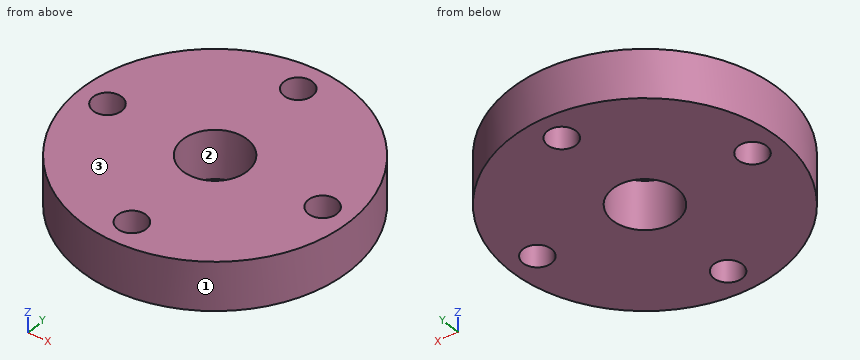
```python
from build123d import *

# Parameters (mm, degrees)
SKETCH1_R           = 16.4
SKETCH1_R_2         = 4
SKETCH1_R_3         = 1.8
BOSS_EXTRUDE1_DEPTH = 6
MOVE_FACE1_BY       = 0.05
MOVE_FACE1_2_BY     = 0.05
MOVE_FACE1_3_BY     = 0.05
MOVE_FACE1_4_BY     = 0.05
MOVE_FACE1_5_BY     = 0.05
MOVE_FACE1_6_BY     = 0.05


with BuildPart() as part:
    # Sketch1 → Boss-Extrude1 (new body)
    with BuildSketch(Plane.XY):
        Circle(SKETCH1_R)
        Circle(SKETCH1_R_2, mode=Mode.SUBTRACT)
        with Locations((0, 13)):
            Circle(SKETCH1_R_3, mode=Mode.SUBTRACT)
        with Locations((13, 0)):
            Circle(SKETCH1_R_3, mode=Mode.SUBTRACT)
        with Locations((0, -13)):
            Circle(SKETCH1_R_3, mode=Mode.SUBTRACT)
        with Locations((-13, 0)):
            Circle(SKETCH1_R_3, mode=Mode.SUBTRACT)
    extrude(amount=BOSS_EXTRUDE1_DEPTH)

    # Move Face1: a curved face moved outward by 0.05
    add(Solid.thicken(part.faces().sort_by_distance((-1.8, 13, 3))[0], MOVE_FACE1_BY))

    # Move Face1 2: a curved face moved outward by 0.05
    add(Solid.thicken(part.faces().sort_by_distance((-16.4, 0, 3))[0], MOVE_FACE1_2_BY))

    # Move Face1 3: a curved face moved outward by 0.05
    add(Solid.thicken(part.faces().sort_by_distance((-4, 0, 3))[0], MOVE_FACE1_3_BY))

    # Move Face1 4: a curved face moved outward by 0.05
    add(Solid.thicken(part.faces().sort_by_distance((11.2, 0, 3))[0], MOVE_FACE1_4_BY))

    # Move Face1 5: a curved face moved outward by 0.05
    add(Solid.thicken(part.faces().sort_by_distance((-1.8, -13, 3))[0], MOVE_FACE1_5_BY))

    # Move Face1 6: a curved face moved outward by 0.05
    add(Solid.thicken(part.faces().sort_by_distance((-14.8, 0, 3))[0], MOVE_FACE1_6_BY))


solid = part.part
```
Design review of the part built by this model. Coordinates are the model's own, in mm. Face numbers are marked on the shaded views. Coordinates: 2 decimals unless noted, no trailing zeros. Order: outer loops, then holes, each group sorted by start corner. A loop starts at its lowest first (then second) coordinate and runs counter-clockwise, first axis right, second up. Notation, with made-up numbers: (-32, 76.5) - (26, 76.5) arc R26 cw to (26, 97.5) - close; hole circle Ø10 at (-29.75, 6.5). An arc over 180 degrees is marked (long way). Answer in a Markdown table with one row per item.
(1) The part is to be moulded in two halves that separate along Y. For the marked faces 1, 2 and 3, say which applies: released by +Y, released by -Y, zero draft, split by the parting line, or undercut.
Checked values:
| item | result |
|---|---|
| face 1 | split by the parting line |
| face 2 | undercut |
| face 3 | zero draft |
(2) Clearance check with flat-ended pins moving along their axes: pin 1 (3 mm diameter, centred on x = 3, y = 3.5, fed in from -Z); pin 2 (1.5 mm diameter, centred on y = -12, z = 4, fed in from -X); pin 3 (3 mm diameter, centred on x = 0, y = 13, fed in from -Z); pin 4 (1.5 mm diameter, centred on x = -10, z = 4, fed in from +Y). State where each tip first meets the part, or that it passes through.
Checked values:
| item | result |
|---|---|
| pin 1 | z = 0 |
| pin 2 | x = -12 |
| pin 3 | through |
| pin 4 | y = 13.6 |
(3) Consider section D-D on x = -13. State the section outline as (y, z) points.
Checked values:
| item | result |
|---|---|
| outline | (-10.08, 0) - (-1.75, 0) - (-1.75, 6) - (-10.08, 6) - close; (1.75, 0) - (10.08, 0) - (10.08, 6) - (1.75, 6) - close |
(4) Consider section A-A on y = 0. State the section outline as (x, z) points, plus the area to 3 significant figures.
Checked values:
| item | result |
|---|---|
| outline | (-16.45, 0) - (-14.75, 0) - (-14.75, 6) - (-16.45, 6) - close; (-11.25, 0) - (-3.95, 0) - (-3.95, 6) - (-11.25, 6) - close; (3.95, 0) - (11.25, 0) - (11.25, 6) - (3.95, 6) - close; (14.75, 0) - (16.45, 0) - (16.45, 6) - (14.75, 6) - close |
| area | 108 mm^2 |
(5) Wall thickness on line 1 along Y through (x, z) = (0, 1.55); line 2 along Y through (x, z) = (1, 3.55); line 3 along Y through (x, z) = (-14, 5.25): over which ranges is each line inside the solid? List them lowest first. Write a range as from..to.
Checked values:
| item | result |
|---|---|
| line 1 | -16.45..-14.75, -11.25..-3.95, 3.95..11.25, 14.75..16.45 |
| line 2 | -16.42..-14.44, -11.56..-3.82, 3.82..11.56, 14.44..16.42 |
| line 3 | -8.64..-1.44, 1.44..8.64 |
(6) Consider section C-C on z = 0.95. State the section outline as (x, y) points, plus the area to 3 significant figures.
Checked values:
| item | result |
|---|---|
| outline | circle Ø32.9 at (0, 0); hole circle Ø3.5 at (-13, 0); hole circle Ø7.9 at (0, 0); hole circle Ø3.5 at (0, -13); hole circle Ø3.5 at (0, 13); hole circle Ø3.5 at (13, 0) |
| area | 763 mm^2 |
